```python
from build123d import *

# Parameters (mm, degrees)
BOSS_EXTRUDE1_DEPTH = 16
SKETCH2_R           = 1.1
CUT_EXTRUDE1_DEPTH  = 2
SKETCH3_R           = 1.5
CUT_EXTRUDE2_DEPTH  = 24
CHAMFER1_SIZE       = 0.8
FILLET1_R           = 2


with BuildPart() as part:
    # Sketch1 → Boss-Extrude1 (new body)
    with BuildSketch(Plane.XY):
        Polygon((0, 0), (0, 8), (3, 8), (3, 2), (23, 2), (23, 0), align=None)
    extrude(amount=BOSS_EXTRUDE1_DEPTH)

    # Sketch2 → Cut-Extrude1 (cut)
    with BuildSketch(Plane(origin=(0, 2, 0), x_dir=(1, 0, 0), z_dir=(0, 1, 0))):
        with Locations((21, -2)):
            Circle(SKETCH2_R)
        with Locations((21, -14)):
            Circle(SKETCH2_R)
    extrude(amount=-CUT_EXTRUDE1_DEPTH, mode=Mode.SUBTRACT)

    # Sketch3 → Cut-Extrude2 (cut, through all)
    with BuildSketch(Plane.ZY):
        with Locations((8, 5.5)):
            Circle(SKETCH3_R)
    extrude(amount=-CUT_EXTRUDE2_DEPTH, mode=Mode.SUBTRACT)

    # Chamfer1
    chamfer1_edges = [part.edges().sort_by_distance(p)[0] for p in [
        (19.9, 2, 2),
        (19.9, 2, 14),
    ]]
    chamfer(chamfer1_edges, length=CHAMFER1_SIZE)

    # Fillet1
    fillet1_edges = [part.edges().sort_by_distance(p)[0] for p in [
        (23, 1, 16),
        (23, 1, 0),
    ]]
    fillet(fillet1_edges, radius=FILLET1_R)


solid = part.part
```
For this review, take the finished solid that the model builds, in its own axes (mm). A direction names the side the tool comes from. Round coordinates to 2 decimals unless told otherwise and drop trailing zeros. Order: outer loops, then holes, each group sorted by start corner. A loop starts at its lowest first (then second) coordinate and runs counter-clockwise, first axis right, second up. Notation, with made-up numbers: (6, 35.25) -> (47, 35.25) arc R3 cw to (47, 40.25) -> close; hole circle Ø8 at (52.5, 31.5). An arc over 180 degrees is marked (long way). Use a Markdown table: item, result.
Item 1: For line 1 along Z through (x, y) = (21, 1); line 2 along X through (y, z) = (0.8, 14); line 3 along Y through (x, z) = (0.65, 8), list the stretches that pass through material, from the lowest coordinate up. Write a range as [from, to].
Resolved:
| item | result |
|---|---|
| line 1 | z = [0, 0.9], [3.1, 12.9], [15.1, 16] |
| line 2 | x = [0, 19.9], [22.1, 23] |
| line 3 | y = [0, 4], [7, 8] |
Item 2: Take a section at B-B (z = 8). State the section outline as (x, y) points.
Resolved:
| item | result |
|---|---|
| outline | (0, 0) -> (23, 0) -> (23, 2) -> (3, 2) -> (3, 4) -> (0, 4) -> close; (0, 7) -> (3, 7) -> (3, 8) -> (0, 8) -> close |
Item 3: For pin 1 (3 mm diameter, centred on y = 6.5, z = 5.5, fed in from +X); pin 2 (5 mm diameter, centred on x = 16, z = 6.5, fed in from +Y); pin 3 (2.5 mm diameter, centred on x = 21, z = 14, fed in from +Y); pin 4 (1.8 mm diameter, centred on y = 5.5, z = 8, fed in from +X), all flat-tipped, find the tip position at first contact; note any pin that passes through.
Resolved:
| item | result |
|---|---|
| pin 1 | stops at x = 3 |
| pin 2 | stops at y = 2 |
| pin 3 | stops at y = 1.35 |
| pin 4 | passes through |
Item 4: Take a section at D-D (z = 5.5). State the section outline as (x, y) points, plus the area to 3 significant figures.
Resolved:
| item | result |
|---|---|
| outline | (0, 0) -> (23, 0) -> (23, 2) -> (3, 2) -> (3, 8) -> (0, 8) -> close |
| area | 64.0 mm² |
Item 5: Machinability: for faces 4 (the flat face through (13, 2, 8)), 5 (the flat face through (1, 8, 8)), which of the approach directions +Z, -Z, +X, -X, +Y, -Y give a long, thin tool a straight path to every point of the face, cutting with its end or side? Answer none if there is none.
Resolved:
| item | result |
|---|---|
| face 4 | +Z, -Z, +X, +Y |
| face 5 | +Z, -Z, +X, -X, +Y |
Item 6: Draft analysis for pull direction X (two halves, no side actions). For faces 1 (the cylindrical face through (19.9, 0.6, 2)), 2 (the cylindrical face through (1.5, 4.6, 6.8)), 3 (the flat face through (0, 3, 8)), state which applies: +X half, -X half, draft (parallel to the pull), parting line (faces both ways), or undercut.
Resolved:
| item | result |
|---|---|
| face 1 | undercut |
| face 2 | draft |
| face 3 | -X half |
Item 7: Take a section at C-C (x = 1.75). State the section outline as (y, z) points.
Resolved:
| item | result |
|---|---|
| outline | (0, 0) -> (8, 0) -> (8, 16) -> (0, 16) -> close; hole circle Ø3 at (5.5, 8) |
Item 8: Take a section at A-A (y = 5.5). State the section outline as (x, z) points.
Resolved:
| item | result |
|---|---|
| outline | (0, 0) -> (3, 0) -> (3, 6.5) -> (0, 6.5) -> close; (0, 9.5) -> (3, 9.5) -> (3, 16) -> (0, 16) -> close |
